Input: part model. Units: mm. Frame: model coordinates. A direction names the side the tool comes from. Coordinates: 2 decimals unless noted, no trailing zeros. Loops run counter-clockwise (first coordinate to the right, second up) from the corner with the lowest first, then second, coordinate; pieces in that order, holes last. Notation, with made-up numbers: (77, -23) - (105, -23) arc R32 ccw to (105, 9) - close; hole circle Ø7 at (66.25, 74.5). An arc over 180 degrees is marked (long way). Use a Markdown table: item, result. Add a question column.
1. Section query C-C on y = 2.5. Return the cut outline in (x, z), then the cut area to 3 significant figures.
2. Section query B-B on z = 0. Return the cut outline in (x, y).
3. Access query for faces 5 (the face through (4, 0.5, 0)), 6 (the face through (11, 0, -4)), 7 (the face through (0, 5, 2)). Directions: +Z, -Z, +X, -X, +Y, -Y. A direction counts if a zero-diameter tool reaches every point of the face in a straight line with its end or side. Return the directions, or none.
4. Draft query along Z for faces 1 (the face through (14.8, 0.5, 3)), 2 (the face through (15.2, 0.5, -3)), 3 (the face through (11.2, 0.5, 8)), 4 (the face through (26, 0.5, 5.5)). Return one class per face: released by +Z, released by -Z, zero draft, split by the parting line, or undercut.
5. Section query D-D on x = 0. Return the cut outline in (y, z).
6. Contact query for flat-ended pins moving along their axis: P1, Ø5, axis at x = 21, z = -3.5, coming from the -Y side; P2, Ø0.5, axis at y = 0.5, z = 0.5, coming from the +X side; P3, Ø1.2, axis at x = 0, z = 0, coming from the +Y side. Output: stop coordinate, or through.
7. Ray query, L1, parallel to X at y = 5, z = 0; L2, parallel to Y at x = 12.25, z = -6. Return the intervals inside material, ascending. Write a range as [from, to].
8. Section query A-A on x = 17.5. Return the cut outline in (y, z), then the cut area to 3 significant figures.
```python
from build123d import *

# Parameters (mm, degrees)
BOSS_EXTRUDE1_DEPTH = 1
SKETCH4_R           = 2
SKETCH4_R_2         = 1
BOSS_EXTRUDE2_DEPTH = 10
CHAMFER1_SIZE       = 0.8


with BuildPart() as part:
    # Sketch3 → Boss-Extrude1 (new body)
    with BuildSketch(Plane(origin=(0, 0, 0), x_dir=(1, 0, 0), z_dir=(0, 1, 0))):
        Polygon((26, 8), (26, 3), (4, 3), (4, -3), (26, -3), (26, -8), (-4, -8), (-4, 8), align=None)
    extrude(amount=BOSS_EXTRUDE1_DEPTH)

    # Sketch4 → Boss-Extrude2 (add)
    with BuildSketch(Plane(origin=(0, 0, 0), x_dir=(1, 0, 0), z_dir=(0, 1, 0))):
        Circle(SKETCH4_R)
        Circle(SKETCH4_R_2, mode=Mode.SUBTRACT)
    extrude(amount=BOSS_EXTRUDE2_DEPTH)

    # Chamfer1
    chamfer1_edges = [part.edges().sort_by_distance(p)[0] for p in [
        (-2, 1, 0),
        (-2, 10, 0),
    ]]
    chamfer(chamfer1_edges, length=CHAMFER1_SIZE)


solid = part.part
```
Resolved:
| question | item | result |
|---|---|---|
| 1 | outline | circle Ø4 at (0, 0); hole circle Ø2 at (0, 0) |
| 1 | area | 9.42 mm² |
| 2 | outline | (-4, 0) - (4, 0) - (4, 1) - (2.8, 1) - (2, 1.8) - (2, 9.2) - (1.2, 10) - (1, 10) - (1, 1) - (-1, 1) - (-1, 10) - (-1.2, 10) - (-2, 9.2) - (-2, 1.8) - (-2.8, 1) - (-4, 1) - close |
| 3 | face 5 | +X, +Y, -Y |
| 3 | face 6 | +Z, -Z, +X, -X, -Y |
| 3 | face 7 | +Y |
| 4 | face 1 | undercut |
| 4 | face 2 | undercut |
| 4 | face 3 | released by +Z |
| 4 | face 4 | zero draft |
| 5 | outline | (0, -8) - (1, -8) - (1, -2.8) - (1.8, -2) - (9.2, -2) - (10, -1.2) - (10, -1) - (1, -1) - (1, 1) - (10, 1) - (10, 1.2) - (9.2, 2) - (1.8, 2) - (1, 2.8) - (1, 8) - (0, 8) - close |
| 6 | P1 | y = 0 |
| 6 | P2 | x = 4 |
| 6 | P3 | y = 1 |
| 7 | L1 | [-2, -1], [1, 2] |
| 7 | L2 | [0, 1] |
| 8 | outline | (0, -8) - (1, -8) - (1, -3) - (0, -3) - close; (0, 3) - (1, 3) - (1, 8) - (0, 8) - close |
| 8 | area | 10.0 mm² |
